Here's the drawing with two shaded views (mm, measured from the low corner). I have some questions. Round coordinates to 2 decimals unless told otherwise and drop trailing zeros. Order: outer loops, then holes, each group sorted by start corner. A loop starts at its lowest first (then second) coordinate and runs counter-clockwise, first axis right, second up.
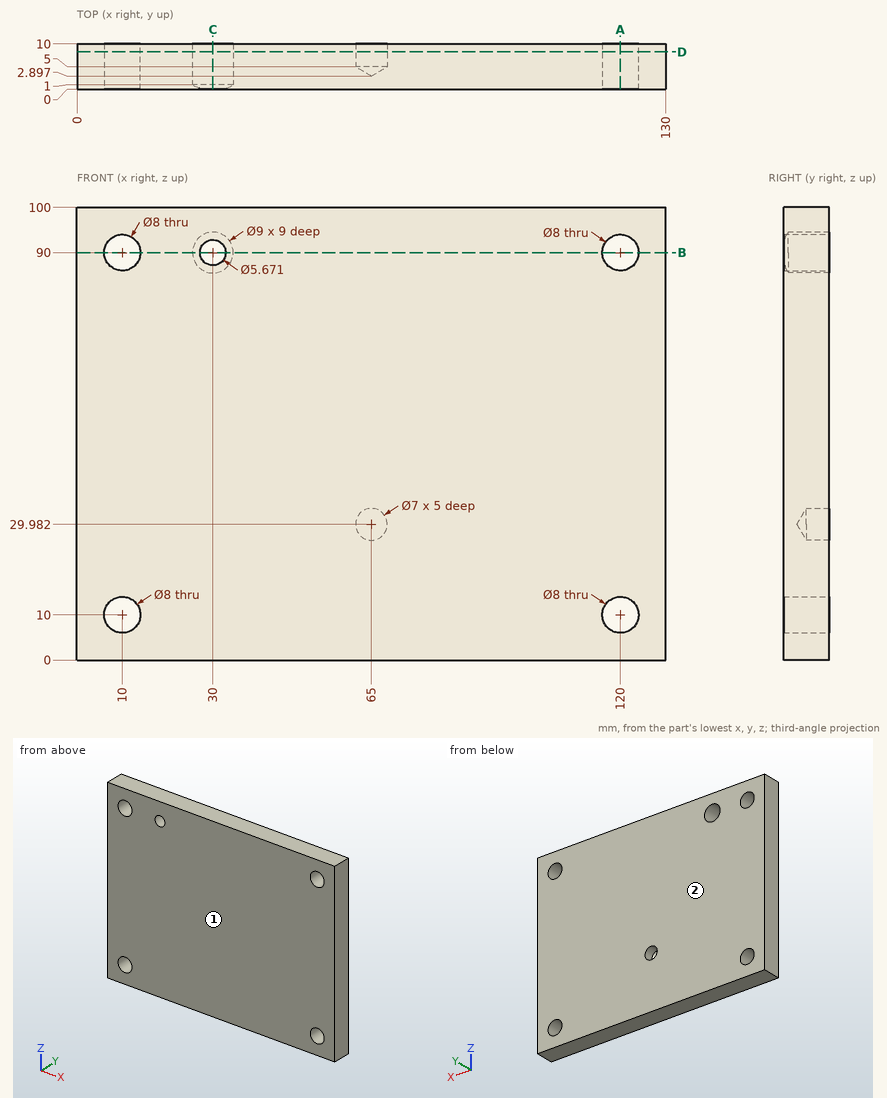
1. I'm going to push flat-ended pins straight in: P1, Ø6.5, axis at x = 120, z = 10, coming from the -Y side (3 decimals); P2, Ø8, axis at x = 30, z = 90, coming from the +Y side. Where does each tip first touch, or does it pass through?
Evaluation:
P1: passes through
P2: stops at y = 0.7
2. If we section it at D-D, the plane y = 8.25: Write out the boundary of the cut face in (x, z).
Evaluation:
outline: (0, 0) - (130, 0) - (130, 100) - (0, 100) - close; hole circle Ø8 at (10, 10); hole circle Ø8 at (10, 90); hole circle Ø9 at (30, 90); hole circle Ø7 at (65, 29.98); hole circle Ø8 at (120, 10); hole circle Ø8 at (120, 90)
3. If we section it at A-A, the plane x = 120: Write out the boundary of the cut face in (y, z), and give its area (3 significant figures).
Evaluation:
outline: (0, 0) - (10, 0) - (10, 6) - (0, 6) - close; (0, 14) - (10, 14) - (10, 86) - (0, 86) - close; (0, 94) - (10, 94) - (10, 100) - (0, 100) - close
area: 840 mm2
4. If we section it at B-B, the plane z = 90: Write out the boundary of the cut face in (x, y) (1 decimal), and give its area (3 significant figures).
Evaluation:
outline: (0, 0) - (6, 0) - (6, 10) - (0, 10) - close; (14, 0) - (27.2, 0) - (25.5, 1) - (25.5, 10) - (14, 10) - close; (32.8, 0) - (116, 0) - (116, 10) - (34.5, 10) - (34.5, 1) - close; (124, 0) - (130, 0) - (130, 10) - (124, 10) - close
area: 1,050 mm2
5. If we mould it in two halves opening along Y, with no side actions, what happens to the marked faces 1 and 2? For each: released by +Y, released by -Y, zero draft, split by the parting line, or undercut.
Evaluation:
face 1: released by -Y
face 2: released by +Y
6. If we section it at C-C, the plane x = 30: Write out the boundary of the cut face in (y, z) (1 decimal).
Evaluation:
outline: (0, 0) - (10, 0) - (10, 85.5) - (1, 85.5) - (0, 87.2) - close; (0, 92.8) - (1, 94.5) - (10, 94.5) - (10, 100) - (0, 100) - close
7. I need wall thicknesses on probe 1 along Z at (x, y) = (10, 4.25); probe 2 along Z at (x, y) = (30, 4.5); probe 3 along Z at (x, y) = (65, 7.05). Which ranges of each line are inside material? Lowest first, please.
Evaluation:
probe 1: z = 0 to 6, 14 to 86, 94 to 100
probe 2: z = 0 to 85.5, 94.5 to 100
probe 3: z = 0 to 26.48, 33.48 to 100
